The listing builds one solid part. Answer for the finished solid, in the listing's coordinates (mm). A direction names the side the tool comes from. Coordinates: 2 decimals unless noted, no trailing zeros. Order: outer loops, then holes, each group sorted by start corner. A loop starts at its lowest first (then second) coordinate and runs counter-clockwise, first axis right, second up. Notation, with made-up numbers: (66, 42.25) -> (109, 42.25) arc R24 cw to (109, 57.25) -> close; hole circle Ø5 at (5, 57.5). An arc over 180 degrees is marked (long way). Return JSON: item names as keys, results as strings.
```python
from build123d import *

# Parameters (mm, degrees)
SKETCH2_W               = 62
SKETCH2_H               = 74
BASE_FLANGE1_DEPTH      = 0.5
CUT_EXTRUDE1_REACH      = 50.273
SKETCH5_R               = 2
SKETCH5_R_2             = 1.6
EDGE_FLANGE1_DEPTH      = 57
EDGE_FLANGE1_BEND_DEPTH = 57
EDGE_FLANGE2_DEPTH      = 69
EDGE_FLANGE2_BEND_DEPTH = 69
BREAK_CORNER1_START     = -32.2366
BREAK_CORNER1_DEPTH     = 64.4732
BREAK_CORNER1_START_2   = -38.2366
BREAK_CORNER1_2_DEPTH   = 76.4732
BREAK_CORNER1_START_3   = -0.5
BREAK_CORNER1_3_DEPTH   = 0.5


# Read off the part's stored shape, not the designer's step: Break-Corner1
# Sheet-metal steps are written as plain solids
with BuildPart() as part:
    # Sketch2 → Base-Flange1 (new body)
    with BuildSketch(Plane(origin=(0, 0, 0), x_dir=(1, 0, 0), z_dir=(0, 1, 0))):
        Rectangle(SKETCH2_W, SKETCH2_H)
    extrude(amount=-BASE_FLANGE1_DEPTH)

    # Sketch5 → Cut-Extrude1 (cut, up to next)
    with BuildSketch(Plane(origin=(0, 0, 0), x_dir=(1, 0, 0), z_dir=(0, 1, 0)), mode=Mode.PRIVATE) as cut_extrude1_sk1:
        with Locations(Location((-26, -32.5, 0), (0, 0, 270))):
            Circle(SKETCH5_R)
    cut_extrude1_tool1 = extrude(cut_extrude1_sk1.sketch, amount=-CUT_EXTRUDE1_REACH, mode=Mode.PRIVATE) & part.part
    # Sketch5 → Cut-Extrude1 (cut, up to next)
    with BuildSketch(Plane(origin=(0, 0, 0), x_dir=(1, 0, 0), z_dir=(0, 1, 0)), mode=Mode.PRIVATE) as cut_extrude1_sk2:
        with Locations(Location((25.2, -15.3, 0), (0, 0, 270))):
            Circle(SKETCH5_R_2)
    cut_extrude1_tool2 = extrude(cut_extrude1_sk2.sketch, amount=-CUT_EXTRUDE1_REACH, mode=Mode.PRIVATE) & part.part
    # Sketch5 → Cut-Extrude1 (cut, up to next)
    with BuildSketch(Plane(origin=(0, 0, 0), x_dir=(1, 0, 0), z_dir=(0, 1, 0)), mode=Mode.PRIVATE) as cut_extrude1_sk3:
        with Locations(Location((-25.6, 0, 0), (0, 0, 270))):
            Circle(SKETCH5_R_2)
    cut_extrude1_tool3 = extrude(cut_extrude1_sk3.sketch, amount=-CUT_EXTRUDE1_REACH, mode=Mode.PRIVATE) & part.part
    # Sketch5 → Cut-Extrude1 (cut, up to next)
    with BuildSketch(Plane(origin=(0, 0, 0), x_dir=(1, 0, 0), z_dir=(0, 1, 0)), mode=Mode.PRIVATE) as cut_extrude1_sk4:
        with Locations(Location((26.8, 33, 0), (0, 0, 270))):
            Circle(SKETCH5_R_2)
    cut_extrude1_tool4 = extrude(cut_extrude1_sk4.sketch, amount=-CUT_EXTRUDE1_REACH, mode=Mode.PRIVATE) & part.part
    # Sketch5 → Cut-Extrude1 (cut, up to next)
    with BuildSketch(Plane(origin=(0, 0, 0), x_dir=(1, 0, 0), z_dir=(0, 1, 0)), mode=Mode.PRIVATE) as cut_extrude1_sk5:
        with Locations(Location((26, -32.5, 0), (0, 0, 270))):
            Circle(SKETCH5_R)
    cut_extrude1_tool5 = extrude(cut_extrude1_sk5.sketch, amount=-CUT_EXTRUDE1_REACH, mode=Mode.PRIVATE) & part.part
    add(cut_extrude1_tool1.solids().sort_by_distance((-26, 0, 32.5))[0], mode=Mode.SUBTRACT)
    add(cut_extrude1_tool2.solids().sort_by_distance((25.2, 0, 15.3))[0], mode=Mode.SUBTRACT)
    add(cut_extrude1_tool3.solids().sort_by_distance((-25.6, 0, 0))[0], mode=Mode.SUBTRACT)
    add(cut_extrude1_tool4.solids().sort_by_distance((26.8, 0, -33))[0], mode=Mode.SUBTRACT)
    add(cut_extrude1_tool5.solids().sort_by_distance((26, 0, 32.5))[0], mode=Mode.SUBTRACT)

    # Edge-Flange1 section (across the edge) → Edge-Flange1 (add)
    with BuildSketch(Plane(origin=(28.5, 0, -37.7366), x_dir=(0, 0, 1), z_dir=(-1, 0, 0))):
        with BuildLine():
            Line((-0.5, 0.7366), (-0.5, 5))
            Line((-0.5, 5), (0, 5))
            Line((0, 5), (0, 0.7366))
            ThreePointArc((0, 0.7366), (0.215745145, 0.215745145), (0.7366, 0))
            Line((0.7366, 0), (0.7366, -0.5))
            ThreePointArc((0.7366, -0.5), (-0.137808246, -0.137808246), (-0.5, 0.7366))
        make_face()
    extrude(amount=EDGE_FLANGE1_DEPTH)

    # Edge-Flange1 section 2 (across the edge) → Edge-Flange1 bend (add)
    with BuildSketch(Plane(origin=(-28.5, 0, 37.7366), x_dir=(0, 0, -1), z_dir=(1, 0, 0))):
        with BuildLine():
            Line((-0.5, 0.7366), (-0.5, 5))
            Line((-0.5, 5), (0, 5))
            Line((0, 5), (0, 0.7366))
            ThreePointArc((0, 0.7366), (0.215745145, 0.215745145), (0.7366, 0))
            Line((0.7366, 0), (0.7366, -0.5))
            ThreePointArc((0.7366, -0.5), (-0.137808246, -0.137808246), (-0.5, 0.7366))
        make_face()
    extrude(amount=EDGE_FLANGE1_BEND_DEPTH)

    # Edge-Flange2 section (across the edge) → Edge-Flange2 (add)
    with BuildSketch(Plane(origin=(31.7366, -0.5, -34.5), x_dir=(-1, 0, 0), z_dir=(0, 0, 1))):
        with BuildLine():
            Line((-0.5, 0.7366), (-0.5, 5))
            Line((-0.5, 5), (0, 5))
            Line((0, 5), (0, 0.7366))
            ThreePointArc((0, 0.7366), (0.215745145, 0.215745145), (0.7366, 0))
            Line((0.7366, 0), (0.7366, -0.5))
            ThreePointArc((0.7366, -0.5), (-0.137808246, -0.137808246), (-0.5, 0.7366))
        make_face()
    extrude(amount=EDGE_FLANGE2_DEPTH)

    # Edge-Flange2 section 2 (across the edge) → Edge-Flange2 bend (add)
    with BuildSketch(Plane(origin=(-31.7366, -0.5, 34.5), x_dir=(1, 0, 0), z_dir=(0, 0, -1))):
        with BuildLine():
            Line((-0.5, 0.7366), (-0.5, 5))
            Line((-0.5, 5), (0, 5))
            Line((0, 5), (0, 0.7366))
            ThreePointArc((0, 0.7366), (0.215745145, 0.215745145), (0.7366, 0))
            Line((0.7366, 0), (0.7366, -0.5))
            ThreePointArc((0.7366, -0.5), (-0.137808246, -0.137808246), (-0.5, 0.7366))
        make_face()
    extrude(amount=EDGE_FLANGE2_BEND_DEPTH)

    # Break-Corner1 outline → Break-Corner1 (cut)
    with BuildSketch(Plane.YZ.offset(BREAK_CORNER1_START)):
        with BuildLine():
            Line((-5.5, 34.5), (-5.5, 32.25))
            ThreePointArc((-5.5, 32.25), (-4.840990258, 33.840990258), (-3.25, 34.5))
            Line((-3.25, 34.5), (-5.5, 34.5))
        make_face()
        with BuildLine():
            ThreePointArc((-3.25, -34.5), (-4.840990258, -33.840990258), (-5.5, -32.25))
            Line((-5.5, -32.25), (-5.5, -34.5))
            Line((-5.5, -34.5), (-3.25, -34.5))
        make_face()
    extrude(amount=BREAK_CORNER1_DEPTH, mode=Mode.SUBTRACT)

    # Break-Corner1 2 outline → Break-Corner1 2 (cut)
    with BuildSketch(Plane.XY.offset(BREAK_CORNER1_START_2)):
        with BuildLine():
            ThreePointArc((-28.5, 2.75), (-27.840990258, 4.340990258), (-26.25, 5))
            Line((-26.25, 5), (-28.5, 5))
            Line((-28.5, 5), (-28.5, 2.75))
        make_face()
        with BuildLine():
            ThreePointArc((26.25, 5), (27.840990258, 4.340990258), (28.5, 2.75))
            Line((28.5, 2.75), (28.5, 5))
            Line((28.5, 5), (26.25, 5))
        make_face()
    extrude(amount=BREAK_CORNER1_2_DEPTH, mode=Mode.SUBTRACT)

    # Break-Corner1 3 outline → Break-Corner1 3 (cut)
    with BuildSketch(Plane(origin=(0, 0, 0), x_dir=(1, 0, 0), z_dir=(0, 1, 0)).offset(BREAK_CORNER1_START_3)):
        with BuildLine():
            ThreePointArc((-28.75, -37), (-30.340990258, -36.340990258), (-31, -34.75))
            Line((-31, -34.75), (-31, -37))
            Line((-31, -37), (-28.75, -37))
        make_face()
        with BuildLine():
            ThreePointArc((-31, 34.75), (-30.340990258, 36.340990258), (-28.75, 37))
            Line((-28.75, 37), (-31, 37))
            Line((-31, 37), (-31, 34.75))
        make_face()
        with BuildLine():
            ThreePointArc((28.75, 37), (30.340990258, 36.340990258), (31, 34.75))
            Line((31, 34.75), (31, 37))
            Line((31, 37), (28.75, 37))
        make_face()
        with BuildLine():
            ThreePointArc((31, -34.75), (30.340990258, -36.340990258), (28.75, -37))
            Line((28.75, -37), (31, -37))
            Line((31, -37), (31, -34.75))
        make_face()
    extrude(amount=BREAK_CORNER1_3_DEPTH, mode=Mode.SUBTRACT)


solid = part.part
```
Item 1: The part is cut by section B-B on x = -13.5. Determine the outline of the cut face in (y, z), plus the area to 3 significant figures.
Answer list:
{"outline": "(-0.5, -37) arc R1.24 ccw to (0.74, -38.24) -> (5, -38.24) -> (5, -37.74) -> (0.74, -37.74) arc R0.74 cw to (0, -37) -> (0, 37) arc R0.74 cw to (0.74, 37.74) -> (5, 37.74) -> (5, 38.24) -> (0.74, 38.24) arc R1.24 ccw to (-0.5, 37) -> close", "area": "42.8 mm2"}
Item 2: The part is cut by section A-A on z = 3.5. Determine the outline of the cut face in (x, y), plus the area to 3 significant figures.
Answer list:
{"outline": "(-32.24, -5.5) -> (-31.74, -5.5) -> (-31.74, -1.24) arc R0.74 cw to (-31, -0.5) -> (31, -0.5) arc R0.74 cw to (31.74, -1.24) -> (31.74, -5.5) -> (32.24, -5.5) -> (32.24, -1.24) arc R1.24 ccw to (31, 0) -> (-31, 0) arc R1.24 ccw to (-32.24, -1.24) -> close", "area": "36.8 mm2"}
Item 3: Find the intervals of material crossed by probe 1 along Z at (x, y) = (-24, 0.75); probe 2 along X at (y, z) = (-3.75, 1); probe 3 along X at (y, z) = (-0.3, 32.5), in increasing order.
Answer list:
{"probe 1": "-38.24 to -37.74, 37.74 to 38.24", "probe 2": "-32.24 to -31.74, 31.74 to 32.24", "probe 3": "-31.81 to -28, -24 to 24, 28 to 31.81"}
Item 4: Which of the six approach directions +Z, -Z, +X, -X, +Y, -Y give full straight-line access (tool end or side, diameter ignored) to faces 1 (the flat face through (-32.237, -3, 0)), 2 (the flat face through (-31.737, -3, 0))?
Answer list:
{"face 1": "+Z, -Z, -X, +Y, -Y", "face 2": "+Z, -Z, -Y"}
Item 5: Determine the mould class of faces 3 (the flat face through (31.737, -3, 0)), 4 (the cylindrical face through (-31.99, -4.86, 33.82)), 5 (the cylindrical face through (-26.766, -0.246, 34.347)) for opening direction Z: pulls with the +Z half, pulls with the -Z half, needs draft (parallel to the pull), parting line crosses it, or undercut.
Answer list:
{"face 3": "needs draft", "face 4": "pulls with the +Z half", "face 5": "undercut"}
Item 6: Flat-ended cylindrical pins translate along their axes: pin 1 (18.5 mm diameter, centred on x = 7.5, z = 14, fed in from +Y); pin 2 (1 mm diameter, centred on y = 0.5, z = -38, fed in from -X); pin 3 (1.4 mm diameter, centred on x = 31.5, y = -2, fed in from -Z). Find the tip coordinate at first contact, or state that the pin passes through.
Answer list:
{"pin 1": "y = 0", "pin 2": "x = -28.5", "pin 3": "z = -34.5"}
